Part model, mm, in its own coordinate system. Face numbers are marked on the shaded views. A direction names the side the tool comes from. Give positions to 0.01 mm unless a question says otherwise; leave off trailing zeros. Write each loop counter-clockwise with the first axis right and the second up, starting at its lowest first coordinate (ties: lowest second). Pieces come first, ordered by that corner, then holes.
Autodesk Fusion 360 part; units mm, degrees
sketch "Sketch1" plane through (0, 0, 0) normal (0, 0, 1) x (1, 0, 0)
  line L0 (36, 27) -> (-36, 27)
  line L1 (-36, 27) -> (-36, -27)
  line L2 (-36, -27) -> (36, -27)
  line L3 (36, -27) -> (36, 27)
  line L4 (36, 30.6) -> (-36, 30.6)
  line L5 (-36, 35.6) -> (-36, -30.6)
  line L6 (-36, -30.6) -> (36, -30.6)
  line L7 (36, -30.6) -> (36, 30.6)
  line L8 (33, 35.6) -> (-36, 35.6)
  line L9 (41, -27.6) -> (41, 27.6)
  line L10 (33, -35.6) -> (-36, -35.6)
  line L11 (-36, -35.6) -> (-36, 30.6)
  arc A0 (41, 27.6) -> (33, 35.6) centre (33, 27.6) ccw
  arc A1 (33, -35.6) -> (41, -27.6) centre (33, -27.6) ccw
  circle A2 centre (-20, 0) radius 1.75
  circle A3 centre (15, 0) radius 1.75
  line L12 (-20, 9.5) -> (15, 9.5)
  arc A4 (15, 9.5) -> (15, 17.5) centre (15, 13.5) ccw
  line L13 (15, 17.5) -> (-20, 17.5)
  arc A5 (-20, 17.5) -> (-20, 9.5) centre (-20, 13.5) ccw
  line L14 (-20, 13.5) -> (15, 13.5) construction
  line L15 (1.75, 0) -> (22.5, 0)
  line L16 (-20, -9.5) -> (15, -9.5)
  line L17 (15, -17.5) -> (-20, -17.5)
  arc A6 (15, -17.5) -> (15, -9.5) centre (15, -13.5) ccw
  arc A7 (-20, -9.5) -> (-20, -17.5) centre (-20, -13.5) ccw
  dimension "d1" = 72
  dimension "d2" = 54
  dimension "d3" = 61.2
  dimension "d6" = 8
  dimension "d32" = 3.5
  dimension "d33" = 3.5
  dimension "d34" = 8
extrude "Extrude1" add sketch "Sketch1" along normal blind 6.4 contours L3 L4 L5 L6 L7 L8 L9 L10 L11 A0 A1 | L0 L4 L5 L7 L11 | L2 L5 L6 L7 L11
extrude "Extrude2" add sketch "Sketch1" along normal blind 24 contours L3 L4 L5 L6 L7 L8 L9 L10 L11 A0 A1
extrude "Extrude3" add sketch "Sketch1" along normal blind 27 and the other way blind -24
sketch "Sketch2" plane through (0, -35.6, 0) normal (0, -1, 0) x (1, 0, 0)
  line L0 (-36, 0) -> (33, 0)
  line L1 (33, 0) -> (33, 27)
  line L2 (-36, 27) -> (-36, 0)
  line L3 (-36, 0) -> (-49.5029, 27)
  line L4 (-36, 0) -> (-6, 0) construction
  line L5 (-36, 27) -> (-49.5029, 27)
  line L6 (33, 27) -> (-36, 27)
  line L7 (-36, 27) -> (-36, 24)
  line L8 (-36, 24) -> (-36.4845, 24)
  line L9 (-36.4845, 24) -> (-48.0026, 24)
  line L10 (-36, 0) -> (-36, 6.4)
  line L11 (-36, 6.4) -> (-36, 6)
  line L12 (-36, 6.4) -> (-39.2007, 6.4)
  line L13 (-36, 0) -> (-32.4, 0)
  line L14 (-49.5029, 27) -> (-47.5029, 27)
  line L15 (-36, 6.4) -> (-32.4, 6.4)
  line L16 (-32.4, 6.4) -> (-32.4, 0)
  dimension "d11" = 116.57
  dimension "d25" = 6.4
  dimension "d36" = 3.6
  dimension "d37" = 2
extrude "Extrude4" add sketch "Sketch2" against normal blind 5 contours L2 L3 L10 L11 L12 | L2 L3 L8 L9 L12
extrude "Extrude5" add sketch "Sketch2" along normal blind -71.2 and the other way blind 66.2 contours L2 L3 L10 L11 L12 | L2 L3 L8 L9 L12
extrude "Extrude6" add sketch "Sketch2" against normal blind 71.2 contours L2 L3 L5 L7 L8 L9 L14
extrude "Extrude7" cut sketch "Sketch2" along normal blind -8.6 and the other way blind 5 contours L0 L2 L10 L11 L13 L15 L16
extrude "Extrude8" cut sketch "Sketch2" along normal blind -66.2 and the other way blind 62.6 contours L0 L2 L10 L11 L13 L15 L16
chamfer "Chamfer1" distance 1 angle 45 2 edges at (-21.6316, 0.6328, 24) (13.3684, 0.6328, 24)
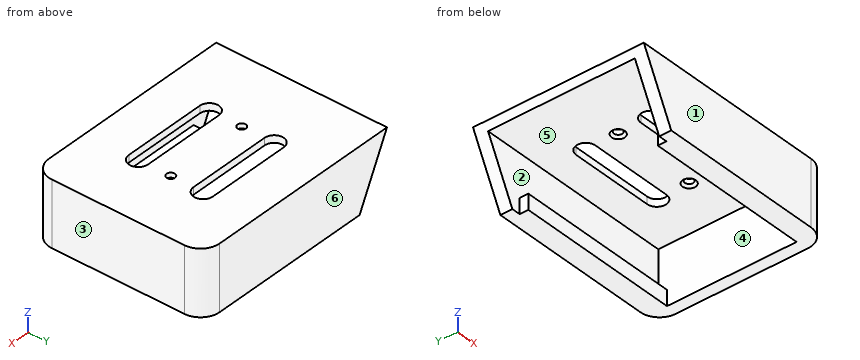
1) Two-plate mould, pull along Y, no slides. Class the marked faces 3, 4, 5 and 6: +Y half, -Y half, draft (parallel to the pull), parting line (faces both ways), or undercut.
Answers follow:
face 3: draft
face 4: undercut
face 5: undercut
face 6: +Y half
2) Saw through at B-B, the plane y = -13.5. Write the cut outline in (x, z), then the cut area to 3 significant figures.
Answers follow:
outline: (-49.5, 27) - (-48, 24) - (-24, 24) - (-24, 27) - close; (19, 24) - (36, 24) - (36, 0) - (41, 0) - (41, 27) - (19, 27) - close
area: 260 mm2
3) Saw through at A-A, the plane x = -11. Write the cut outline in (y, z).
Answers follow:
outline: (-35.6, 0) - (-27, 0) - (-27, 6.4) - (-30.6, 6.4) - (-30.6, 24) - (-17.5, 24) - (-17.5, 27) - (-35.6, 27) - close; (-9.5, 24) - (9.5, 24) - (9.5, 27) - (-9.5, 27) - close; (17.5, 24) - (30.6, 24) - (30.6, 6.4) - (27, 6.4) - (27, 0) - (35.6, 0) - (35.6, 27) - (17.5, 27) - close
4) Saw through at C-C, the plane z = 14.5. Write the cut outline in (x, y), then the cut area to 3 significant figures.
Answers follow:
outline: (-43.25, -35.6) - (33, -35.6) arc R8 ccw to (41, -27.6) - (41, 27.6) arc R8 ccw to (33, 35.6) - (-43.25, 35.6) - (-43.25, 30.6) - (36, 30.6) - (36, -30.6) - (-43.25, -30.6) - close
area: 1,120 mm2
5) Saw through at D-D, the plane x = -28. Write the cut outline in (y, z), then the cut area to 3 significant figures.
Answers follow:
outline: (-35.6, 0) - (-27, 0) - (-27, 6.4) - (-30.6, 6.4) - (-30.6, 24) - (30.6, 24) - (30.6, 6.4) - (27, 6.4) - (27, 0) - (35.6, 0) - (35.6, 27) - (-35.6, 27) - close
area: 500 mm2
6) Wall check: L1, parallel to Y at x = 15, z = 26.6; L2, parallel to Y at x = -4, z = 24.5; L3, parallel to Y at x = -20.5, z = 9.5. Give the ranges that are in metal, low to high.
Answers follow:
L1: y = -35.6 to -17.5, -9.5 to -1.75, 1.75 to 9.5, 17.5 to 35.6
L2: y = -35.6 to -17.5, -9.5 to 9.5, 17.5 to 35.6
L3: y = -35.6 to -30.6, 30.6 to 35.6
7) 3-axis set-ups, long thin cutter, end or side, ignore diameter. For the marked faces 1 and 2: which of +Z, -Z, +X, -X, +Y, -Y reach the whole face in a straight line?
Answers follow:
face 1: +Z, -Z, +X, -X, -Y
face 2: -X
8) Pin check, flat tips, straight feed: pin 1 Ø1.8 at (y, z) = (-29.5, 2.5) entering from -X; pin 2 Ø3 at (x, y) = (6, -21.5) entering from -Z; pin 3 Ø4 at (x, y) = (15, 0) entering from -Z. Stop position of each tip, or through.
Answers follow:
pin 1: stops at x = -32.4
pin 2: stops at z = 24
pin 3: stops at z = 24.75
